Autodesk Inventor part; units mm, degrees
ref_plane "YZ Plane" through (0, 0, 0) normal (1, 0, 0) x (0, 1, 0)
ref_plane "XZ Plane" through (0, 0, 0) normal (0, 1, 0) x (-1, 0, 0)
ref_plane "XY Plane" through (0, 0, 0) normal (0, 0, 1) x (1, 0, 0)
sketch "Sketch1" plane through (0, 0, 0) normal (1, 0, 0) x (0, 1, 0)
  line L0 (-90, 74.5) -> (90, 74.5)
  line L1 (90, 74.5) -> (90, -74.5)
  line L2 (90, -74.5) -> (-90, -74.5)
  line L3 (-90, -74.5) -> (-90, 74.5) construction
  line L4 (-90, 74.5) -> (90, -74.5) construction
  line L5 (90, 74.5) -> (-90, -74.5) construction
  line L6 (85, 74.5) -> (85, 46.75)
  line L7 (85, 46.75) -> (90, 46.75)
  line L8 (0, 74.5) -> (0, -74.5)
  line L9 (90, 0) -> (-90, 0) construction
  arc A0 (85, 49.75) -> (85, 46.75) centre (85, 48.25) ccw
  line L10 (-90, 74.5) -> (-90, -74.5)
  circle A1 centre (73, 65) radius 3 construction
  arc A2 (73, 67.1) -> (73, 62.9) centre (73, 65) ccw construction
  line L11 (73, 67.1) -> (76.5201, 67.1) construction
  arc A3 (76.5201, 62.9) -> (76.5201, 67.1) centre (80.5, 65) ccw construction
  line L12 (73, 65) -> (80.5, 65) construction
  line L13 (73, 62.9) -> (76.5201, 62.9) construction
  line L14 (90, 28.75) -> (85, 28.75) construction
  line L15 (90, 14.75) -> (85, 14.75) construction
  line L16 (90, 21.75) -> (85, 21.75) construction
  line L17 (85, -3.25) -> (90, -3.25)
  arc A4 (85, -3.25) -> (85, -6.25) centre (85, -4.75) ccw
  line L18 (85, -6.25) -> (85, -74.5)
  line L19 (90, -31) -> (-90, -31)
  line L20 (74, -31) -> (74, -74.5)
  line L21 (-90, 21.75) -> (90, 21.75) construction
  circle A5 centre (73, -21.5) radius 3 construction
  arc A6 (73, -19.4) -> (73, -23.6) centre (73, -21.5) ccw construction
  line L22 (73, -23.6) -> (76.5201, -23.6) construction
  arc A7 (76.5201, -23.6) -> (76.5201, -19.4) centre (80.5, -21.5) ccw construction
  line L23 (73, -21.5) -> (80.5, -21.5) construction
  line L24 (73, -19.4) -> (76.5201, -19.4) construction
  arc A8 (74, -31) -> (74, -34) centre (74, -32.5) ccw
  point P0 (0, 0)
  point P1 (90, -3.25)
  point P2 (85, -31)
  point P3 (85, 65)
  point P4 (85, -21.5)
  point P5 (0, -31)
  dimension "d0" = 180
  dimension "d1" = 149
  dimension "d2" = 1.5
  dimension "d3" = 5
  dimension "d15" = 6
  dimension "d16" = 4.2
  dimension "d17" = 9
  dimension "d18" = 5
  dimension "d27" = 5
  dimension "d28" = 14
  dimension "d38" = 50
  dimension "d40" = 52.75
  dimension "d44" = 11
  dimension "d45" = 43.5
  dimension "d46" = 5
  dimension "d47" = 105.5
extrude "Extrusion1" add sketch "Sketch1" along normal blind 5 contours L0 L6 A0 L7 L1 L17 A4 L18 L19 L8 | L19 A8 L20 L2 L8
sketch "Sketch2" plane through (0, 90, 46.75) normal (0, 1, 0) x (1, 0, 0)
  line L0 (5, 32) -> (0, 32) construction
  line L1 (5, 18) -> (0, 18) construction
  line L2 (5, 50) -> (5, 0)
  line L3 (0, 50) -> (0, 0)
  point P0 (0, 46.75)
  point P1 (2.5, 32)
  point P2 (2.5, 18)
  point P3 (0, 18)
  point P4 (0, 32)
  point P5 (5, 121.25)
  point P6 (5, -27.75)
  point P7 (0, 121.25)
  point P8 (0, -27.75)
  point P9 (5, 77.75)
  point P10 (0, 77.75)
hole "Side-M2" at (2.5, 90, 14.75) at (2.5, 90, 28.75) direction (0, -1, 0) diameter 1.567 depth 5
hole "M3" at (0, 73, 65) at (0, 73, -21.5) direction (1, 0, 0) diameter 2.459 end through all
sketch "Sketch3" plane through (0, 85, 74.5) normal (0, 1, 0) x (1, 0, 0)
  line L0 (5, 24.75) -> (5, 0)
  line L1 (5, 17.75) -> (0, 17.75)
  line L2 (5, 105.5) -> (5, 80.75)
  line L3 (5, 87.75) -> (0, 87.75)
  line L4 (0, 24.75) -> (0, 0)
  line L5 (0, 105.5) -> (0, 80.75)
  line L6 (0, 52.75) -> (5, 52.75) construction
  point P0 (0, 74.5)
  point P1 (2.5, 17.75)
  point P2 (2.5, 87.75)
  point P3 (0, 52.75)
  dimension "d48" = 70
hole "Phi3.0" at (2.5, 85, 56.75) at (2.5, 85, -13.25) direction (0, -1, 0) diameter 3 depth 6
chamfer "C0.5" distance 0.5 angle 45 2 edges at (2.5, 90, 46.75) (2.5, 90, -3.25)
mirror "Mirror1" about plane through (0, 0, 0) normal (0, 1, 0)
equation "\"d40\" = 0.5 * d47"
equation "\"d13\" = d27"
properties part number "TorsoCoverFrameBasis" material "Acetal Resin, Black"
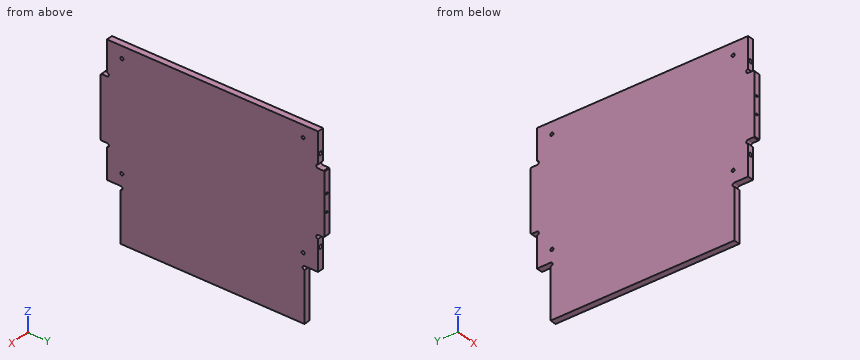
For this review, take the finished solid that the model builds, in its own axes (mm). Round coordinates to 2 decimals unless told otherwise and drop trailing zeros. Use one line per item in the form item = value.
Item 1: For line 1 (Z direction, x = 2.5, y = 87.1); line 2 (Y direction, x = 3.4, z = -21.5); line 3 (Z direction, x = 2.5, y = -82.8), list the stretches that pass through material, from the lowest coordinate up.
Answers:
line_1 = -3.25 to 13.97, 15.53 to 27.97, 29.53 to 46.75
line_2 = -85 to -74.23, -71.77 to 71.77, 74.23 to 85
line_3 = -31 to -14.75, -11.75 to 55.25, 58.25 to 74.5
Item 2: Consider section A-A on x = 2.5. State how many separate pieces and enclosed holes the cut face has, then the cut area to 3 significant figures.
Answers:
separate_pieces = 1
enclosed_holes = 4
area = 24,700 mm^2
Item 3: Clearance check with flat-ended pins moving along their axes: P1, Ø1.3, axis at x = 2.5, z = 29, coming from the -Y side; P2, Ø2, axis at y = -73, z = -21.5, coming from the -X side; P3, Ø1.3, axis at x = 2.5, z = 28.75, coming from the -Y side; P4, Ø1.5, axis at x = 2.5, z = 57, coming from the -Y side. State where each tip first meets the part, or that it passes through.
Answers:
P1 = -90
P2 = through
P3 = -85
P4 = -79
